```python
from build123d import *

# Parameters (mm, degrees)
BOSS_EXTRUDE1_DEPTH             = 5
TAP_DRILL_FOR_M3X0_5_TAP1_D     = 2.5
SKETCH5_W                       = 30
SKETCH5_H                       = 10
BOSS_EXTRUDE2_DEPTH             = 5
FILLET1_R                       = 3
TAP_DRILL_FOR_M3X0_5_TAP2_D     = 2.5
TAP_DRILL_FOR_M3X0_5_TAP2_DEPTH = 5
TAP_DRILL_FOR_M3X0_5_TAP2_TIP   = 0.751075774


with BuildPart() as part:
    # Sketch1 → Boss-Extrude1 (new body)
    with BuildSketch(Plane(origin=(0, 0, 0), x_dir=(1, 0, 0), z_dir=(0, 1, 0))):
        with BuildLine():
            Line((20.955, -43.18), (-20.955, -43.18))
            ThreePointArc((-20.955, -43.18), (-25.445128061, -41.320128061), (-27.305, -36.83))
            Line((-27.305, -36.83), (-27.305, 36.83))
            ThreePointArc((-27.305, 36.83), (-25.445128061, 41.320128061), (-20.955, 43.18))
            Line((-20.955, 43.18), (20.955, 43.18))
            ThreePointArc((20.955, 43.18), (25.445128061, 41.320128061), (27.305, 36.83))
            Line((27.305, 36.83), (27.305, -36.83))
            ThreePointArc((27.305, -36.83), (25.445128061, -41.320128061), (20.955, -43.18))
        make_face()
    extrude(amount=BOSS_EXTRUDE1_DEPTH)

    # Tap Drill for M3x0.5 Tap1 (through all)
    with Locations(Plane(origin=(0, 5, 0), x_dir=(1, 0, 0), z_dir=(0, 1, 0))):
        with Locations((-24.13, 35.345352113), (24.13, 35.345352113), (-20.955, -30.694647887), (20.955, -30.694647887)):
            Hole(TAP_DRILL_FOR_M3X0_5_TAP1_D / 2)

    # Sketch5 → Boss-Extrude2 (add)
    with BuildSketch(Plane(origin=(0, 5, 0), x_dir=(1, 0, 0), z_dir=(0, 1, 0))):
        with Locations((0, 48.18)):
            Rectangle(SKETCH5_W, SKETCH5_H)
    extrude(amount=-BOSS_EXTRUDE2_DEPTH)

    # Fillet1
    fillet1_edges = [part.edges().sort_by_distance(p)[0] for p in [
        (-15, 2.5, -43.18),
        (-15, 2.5, -53.18),
        (15, 2.5, -53.18),
        (15, 2.5, -43.18),
    ]]
    fillet(fillet1_edges, radius=FILLET1_R)

    # Tap Drill for M3x0.5 Tap2
    with Locations(Plane(origin=(0, 0, -53.18), x_dir=(-1, 0, 0), z_dir=(0, 0, -1))):
        with Locations((8, 1.5), (-8, 1.5)):
            Hole(TAP_DRILL_FOR_M3X0_5_TAP2_D / 2, depth=TAP_DRILL_FOR_M3X0_5_TAP2_DEPTH)
            with Locations((0, 0, -(TAP_DRILL_FOR_M3X0_5_TAP2_DEPTH + TAP_DRILL_FOR_M3X0_5_TAP2_TIP / 2))):  # 118° drill point
                Cone(0, TAP_DRILL_FOR_M3X0_5_TAP2_D / 2, TAP_DRILL_FOR_M3X0_5_TAP2_TIP, mode=Mode.SUBTRACT)


solid = part.part
```
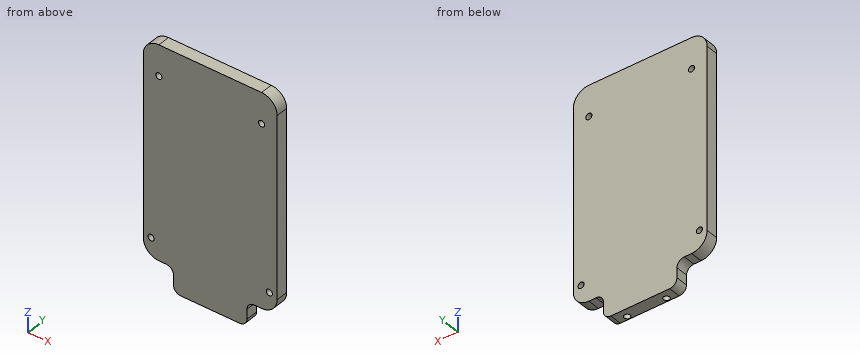
Geometry: final body of the model. Coordinates: model frame, mm. Coordinates: 2 decimals unless noted, no trailing zeros. Order: outer loops, then holes, each group sorted by start corner. A loop starts at its lowest first (then second) coordinate and runs counter-clockwise, first axis right, second up. Notation, with made-up numbers: (19, 47.5) - (59, 47.5) arc R30 cw to (59, 76.5) - close; hole circle Ø1 at (-8.5, 80). An arc over 180 degrees is marked (long way). Write each question's results on one line, items separated by ' | '.
1) Section A-A, the plane y = 3.7. Return loops of the section in (x, z) (3 decimals).
Results list:
outline: (-27.305, -36.83) arc R6.35 ccw to (-20.955, -43.18) - (-18, -43.18) arc R3 cw to (-15, -46.18) - (-15, -50.18) arc R3 ccw to (-12, -53.18) - (12, -53.18) arc R3 ccw to (15, -50.18) - (15, -46.18) arc R3 cw to (18, -43.18) - (20.955, -43.18) arc R6.35 ccw to (27.305, -36.83) - (27.305, 36.83) arc R6.35 ccw to (20.955, 43.18) - (-20.955, 43.18) arc R6.35 ccw to (-27.305, 36.83) - close; hole circle Ø2.5 at (-24.13, -35.345); hole circle Ø2.5 at (-20.955, 30.695); hole circle Ø2.5 at (20.955, 30.695); hole circle Ø2.5 at (24.13, -35.345)
2) Section C-C, the plane x = -24. Return loops of the section in (y, z).
Results list:
outline: (0, -42.4) - (5, -42.4) - (5, -36.59) - (0, -36.59) - close; (0, -34.1) - (5, -34.1) - (5, 42.4) - (0, 42.4) - close
3) Pin query (flat end, axial travel): pin 1 (0.9 mm diameter, centred on x = -19.5, y = 3, fed in from -Z); pin 2 (3 mm diameter, centred on y = 1.5, z = -49, fed in from +X); pin 3 (2 mm diameter, centred on y = 3, z = -49, fed in from -X). Return the tip coordinate at first contact, or that it passes through.
Results list:
pin 1: z = -43.18 | pin 2: x = 15 | pin 3: x = -15
4) Section B-B, the plane x = 24.13. Return loops of the section in (y, z), plus the area to 3 significant figures.
Results list:
outline: (0, -42.33) - (5, -42.33) - (5, -36.6) - (0, -36.6) - close; (0, -34.1) - (5, -34.1) - (5, 42.33) - (0, 42.33) - close | area: 411 mm^2
5) Line query: line 1 (Y direction, x = -8, z = -51.55); line 2 (X direction, y = 1.5, z = -52); line 3 (X direction, y = 3.7, z = -35) (3 decimals). Output: solid intervals per line, ascending. Write a range as from..to.
Results list:
line 1: 0..0.25, 2.75..5 | line 2: -14.38..-9.25, -6.75..6.75, 9.25..14.38 | line 3: -27.305..-25.331, -22.929..22.929, 25.331..27.305
6) Section D-D, the plane x = -16.5. Return loops of the section in (y, z), plus the area to 3 significant figures.
Results list:
outline: (0, -43.58) - (5, -43.58) - (5, 43.18) - (0, 43.18) - close | area: 434 mm^2
